Can you work these out from the model? Positions are in its coordinate system, mm. A direction names the side the tool comes from. Round coordinates to 2 decimals unless told otherwise and drop trailing zeros. Write each loop counter-clockwise with the first axis right and the second up, starting at its lowest first coordinate (ties: lowest second). Pieces come first, ordered by that corner, then holes. Notation, with made-up numbers: (82.5, 15.25) - (131.5, 15.25) arc R4 ccw to (131.5, 19.25) - close; hole circle Ø7 at (-17, 49.5). An arc over 180 degrees is marked (long way). One line per item, written item: value. Start each with the question number.
(1) I'm going to push a flat-ended pin straight in: pin 1 Ø3.5 at (x, y) = (-77.84, 80.72) entering from -Z. Where does the tip first touch, or does it pass through?
(2) On a 3-axis mill with a long thin cutter (end or side, diameter ignored), from which of +Z, -Z, +X, -X, +Y, -Y can I reach the whole of each face in a straight line? I mean faces 4 (the face through (34, 6.721, 2)), 5 (the face through (-59.843, 64, 2)). Say none if no direction works.
(3) I want a section at A-A on x = 121.5. List the corners of the cut face in (y, z) for me.
(4) I want a section at B-B on z = 1.25. Give the number of separate pieces and of enclosed holes in the cut face, plus the area to 3 significant figures.
(5) If I drill on L1, parallel to Y at x = -78, z = 2.8; L2, parallel to Y at x = -34, z = 2.7; L3, parallel to X at y = 28, z = 3.85, over which ranges is the centre line in solid material (lowest first)? Write a range as from..to.
(6) Thinking about a two-plate mould opening in Y: for faces 1 (the face through (-55.843, 47, 2)), 2 (the face through (34, 86.721, 2)), 3 (the face through (161.058, 46, 2)), which applies, +Y half, -Y half, draft (parallel to the pull), parting line (faces both ways), or undercut?
from build123d import *

# Parameters (mm, degrees)
SKETCH_1_W          = 249.901599808
SKETCH_1_H          = 80
EXTRUDE_1_DEPTH     = 4
SKETCH_2_R          = 2.75
SKETCH_2_R_2        = 2.55
CUT_EXTRUDE_1_DEPTH = 4
CUT_EXTRUDE_2_DEPTH = 10
SKETCH_4_R          = 1.6
CUT_EXTRUDE_3_DEPTH = 5
CUT_EXTRUDE_4_DEPTH = 10
FILLET_1_R          = 1.5
SKETCH_6_R          = 1.6
SKETCH_6_R_2        = 2.5
SKETCH_6_R_3        = 11.5
CUT_EXTRUDE_5_DEPTH = 5


with BuildPart() as part:
    # 草图1 → 凸台-拉伸1 (new body)
    with BuildSketch(Plane.XY):
        with Locations((36.107693766, 46.720773392)):
            Rectangle(SKETCH_1_W, SKETCH_1_H)
    extrude(amount=EXTRUDE_1_DEPTH)

    # 草图2 → 切除-拉伸1 (cut)
    with BuildSketch(Plane.XY.offset(4)):
        with Locations((20.45849367, 46.720773392)):
            Circle(SKETCH_2_R)
        with Locations((65.45849367, 46.720773392)):
            Circle(SKETCH_2_R)
        with Locations((42.95849367, 46.720773392)):
            Circle(SKETCH_2_R_2)
    extrude(amount=-CUT_EXTRUDE_1_DEPTH, mode=Mode.SUBTRACT)

    # 草图3 → 切除-拉伸2 (cut)
    with BuildSketch(Plane.XY.offset(4)):
        with BuildLine():
            Line((80.45849367, 68.630603448), (80.45849367, 24.810943336))
            ThreePointArc((80.45849367, 24.810943336), (82.829838109, 20.557689294), (87.694561647, 20.338807381))
            Line((87.694561647, 20.338807381), (131.51422176, 42.248637437))
            ThreePointArc((131.51422176, 42.248637437), (134.278153782, 46.720773392), (131.51422176, 51.192909347))
            Line((131.51422176, 51.192909347), (87.694561647, 73.102739403))
            ThreePointArc((87.694561647, 73.102739403), (82.829838109, 72.88385749), (80.45849367, 68.630603448))
        make_face()
    extrude(amount=-CUT_EXTRUDE_2_DEPTH, mode=Mode.SUBTRACT)

    # 草图4 → 切除-拉伸3 (cut)
    with BuildSketch(Plane.XY.offset(4)):
        with Locations((-77.843106138, 80.720773392)):
            Circle(SKETCH_4_R)
        with Locations((-77.843106138, 68.720773392)):
            Circle(SKETCH_4_R)
        with Locations((-66.843106138, 80.720773392)):
            Circle(SKETCH_4_R)
        with Locations((-66.843106138, 68.720773392)):
            Circle(SKETCH_4_R)
        with Locations((138.05849367, 80.720773392)):
            Circle(SKETCH_4_R)
        with Locations((138.05849367, 68.720773392)):
            Circle(SKETCH_4_R)
        with Locations((148.05849367, 80.720773392)):
            Circle(SKETCH_4_R)
        with Locations((148.05849367, 68.720773392)):
            Circle(SKETCH_4_R)
        with Locations((148.05849367, 24.720773392)):
            Circle(SKETCH_4_R)
        with Locations((148.05849367, 12.720773392)):
            Circle(SKETCH_4_R)
        with Locations((138.05849367, 24.720773392)):
            Circle(SKETCH_4_R)
        with Locations((138.05849367, 12.720773392)):
            Circle(SKETCH_4_R)
        with Locations((-66.843106138, 24.720773392)):
            Circle(SKETCH_4_R)
        with Locations((-66.843106138, 12.720773392)):
            Circle(SKETCH_4_R)
        with Locations((-77.843106138, 24.720773392)):
            Circle(SKETCH_4_R)
        with Locations((-77.843106138, 12.720773392)):
            Circle(SKETCH_4_R)
    extrude(amount=-CUT_EXTRUDE_3_DEPTH, mode=Mode.SUBTRACT)

    # 草图5 → 切除-拉伸4 (cut)
    with BuildSketch(Plane.XY.offset(4)):
        Polygon((-59.843106138, 71.720773392), (-5.115253875, 71.720773392), (-5.115253875, 21.720773392), (-59.843106138, 21.720773392), (-59.843106138, 36.720773392), (-55.843106138, 36.720773392), (-55.843106138, 56.720773392), (-59.843106138, 56.720773392), align=None)
    extrude(amount=-CUT_EXTRUDE_4_DEPTH, mode=Mode.SUBTRACT)

    # 圆角1
    fillet_1_edges = [part.edges().sort_by_distance(p)[0] for p in [
        (-59.843106138, 56.720773392, 2),
        (-59.843106138, 71.720773392, 2),
        (-5.115253875, 71.720773392, 2),
        (-5.115253875, 21.720773392, 2),
        (-59.843106138, 21.720773392, 2),
        (-59.843106138, 36.720773392, 2),
    ]]
    fillet(fillet_1_edges, radius=FILLET_1_R)

    # 草图6 → 切除-拉伸5 (cut)
    with BuildSketch(Plane(origin=(0, 0, 0), x_dir=(-1, 0, 0), z_dir=(0, 0, -1))):
        with Locations((-25.244914522, 56.006736658)):
            Circle(SKETCH_6_R)
        with Locations((-43.773403156, 26.737382225)):
            Circle(SKETCH_6_R)
        with Locations((-59.857163331, 57.418201293)):
            Circle(SKETCH_6_R)
        with Locations((-60.672072817, 37.434810126)):
            Circle(SKETCH_6_R_2)
        with Locations((-42.95849367, 46.720773392)):
            Circle(SKETCH_6_R_3)
    extrude(amount=-CUT_EXTRUDE_5_DEPTH, mode=Mode.SUBTRACT)


solid = part.part
Established:
1. pin 1: z = 0
2. face 4: +Z, -Z, +X, -X, -Y
2. face 5: +Z, -Z
3. outline: (6.72, 0) - (37.24, 0) - (37.24, 4) - (6.72, 4) - close; (56.2, 0) - (86.72, 0) - (86.72, 4) - (56.2, 4) - close
4. separate pieces: 1
4. enclosed holes: 25
4. area: 15,000 mm2
5. L1: 6.72..11.13, 14.31..23.13, 26.31..67.13, 70.31..79.13, 82.31..86.72
5. L2: 6.72..21.72, 71.72..86.72
5. L3: -88.84..-59.84, -5.12..42.79, 44.76..80.46, 103.02..161.06
6. face 1: undercut
6. face 2: +Y half
6. face 3: draft
